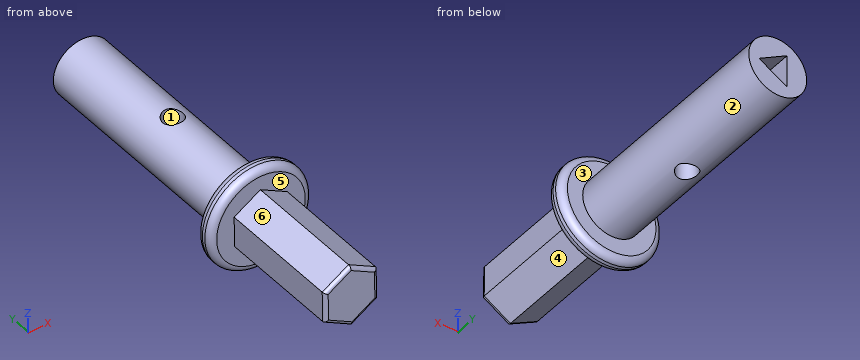
```python
from build123d import *

# Parameters (mm, degrees)
F0_R      = 4.25
F1_DEPTH  = 33
F2_DEPTH  = 6
F3_R      = 7.5
F3_R_2    = 4.25
F4_DEPTH  = 2.5
F6_DEPTH  = 18
F7_R      = 0.5
F8_R      = 1
F10_R     = 1.5
F11_DEPTH = 40


with BuildPart() as f1:
    # F0 (on Front) → F1 (new body)
    with BuildSketch(Plane.XZ):
        Circle(F0_R)
        Polygon((-1.375, 2.38157), (2.75, 0), (-1.375, -2.38157), align=None, mode=Mode.SUBTRACT)
        Polygon((-1.375, -2.38157), (2.75, 0), (-1.375, 2.38157), align=None)
    extrude(amount=F1_DEPTH)

    # F0 (on Front) → F2 (cut)
    with BuildSketch(Plane.XZ):
        Polygon((-1.375, -2.38157), (2.75, 0), (-1.375, 2.38157), align=None)
    extrude(amount=F2_DEPTH, mode=Mode.SUBTRACT)

    # F3 (on face) → F4 (join)
    with BuildSketch(Plane.XZ.offset(33)):
        Circle(F3_R)
        Circle(F3_R_2, mode=Mode.SUBTRACT)
        Circle(F3_R_2)
    extrude(amount=F4_DEPTH)

    # F5 (on face) → F6 (join)
    with BuildSketch(Plane.XZ.offset(35.5)):
        Polygon((0.076423, -4.499351), (3.934764, -2.183492), (3.858341, 2.315859), (-0.076423, 4.499351), (-3.934764, 2.183492), (-3.858341, -2.315859), align=None)
    extrude(amount=F6_DEPTH)

    # F7
    f7_edges = [f1.edges().sort_by_distance(p)[0] for p in [
        (2.005593, -53.5, -3.341421),
        (-1.890959, -53.5, -3.407605),
        (-3.896552, -53.5, -0.066184),
        (-2.005593, -53.5, 3.341421),
        (1.890959, -53.5, 3.407605),
        (3.896552, -53.5, 0.066184),
    ]]
    fillet(f7_edges, radius=F7_R)

    # F8
    f8_edges = [f1.edges().sort_by_distance(p)[0] for p in [
        (-7.5, -35.5, 0),
        (-7.5, -33, 0),
    ]]
    fillet(f8_edges, radius=F8_R)

    # F10 (on offset) → F11 (cut)
    with BuildSketch(Plane.XY.offset(25)):
        with Locations((0, -18)):
            Circle(F10_R)
    extrude(amount=-F11_DEPTH, mode=Mode.SUBTRACT)


solid = f1.part
```
Check sheet for the modelled part. Datum: model origin and axes. Units: mm. Face numbers are marked on the shaded views. A direction names the side the tool comes from. Coordinates: 2 decimals unless noted, no trailing zeros. Write each loop counter-clockwise with the first axis right and the second up, starting at its lowest first coordinate (ties: lowest second). Pieces come first, ordered by that corner, then holes. Notation, with made-up numbers: (-3, -12) -> (8, -12) arc R34 cw to (8, 22) -> close; hole circle Ø3 at (52, -15). An arc over 180 degrees is marked (long way). Use a Markdown table: item, result.
1. Sectioned sample at C-C (y = -8). Enter the section's corners in (x, z), plus the area to 3 significant figures.
Reported:
| item | result |
|---|---|
| outline | circle Ø8.5 at (0, 0) |
| area | 56.7 mm2 |
2. Release check for a two-part mould opening along X. For the marked faces 1, 2 and 3 record: pulls with the +X half, pulls with the -X half, needs draft (parallel to the pull), parting line crosses it, or undercut.
Reported:
| item | result |
|---|---|
| face 1 | undercut |
| face 2 | parting line crosses it |
| face 3 | needs draft |
3. Tool access check on the marked faces 4, 5 and 6. Record the directions out of +Z, -Z, +X, -X, +Y, -Y that give a thin tool (end or side, any length) a straight path to the whole face; none if there is none.
Reported:
| item | result |
|---|---|
| face 4 | -Z, +X, -Y |
| face 5 | -Y |
| face 6 | +Z, -X, -Y |
4. Go/stop test with flat-tipped pins: pin 1 Ø1 at (y, z) = (-31.5, 2) entering from +X; pin 2 Ø6 at (y, z) = (-23.5, 1) entering from +X; pin 3 Ø8 at (x, y) = (4.5, -33.5) entering from +Z; pin 4 Ø2 at (x, z) = (1.5, 0) entering from +Y. Record where each tip stops, or that it passes through.
Reported:
| item | result |
|---|---|
| pin 1 | stops at x = 3.98 |
| pin 2 | stops at x = 4.25 |
| pin 3 | stops at z = 7.48 |
| pin 4 | stops at y = 0 |
5. Sectioned sample at A-A (y = -42). Enter the section's corners in (x, z), plus the area to 3 significant figures.
Reported:
| item | result |
|---|---|
| outline | (-3.93, 2.18) -> (-3.86, -2.32) -> (0.08, -4.5) -> (3.93, -2.18) -> (3.86, 2.32) -> (-0.08, 4.5) -> close |
| area | 52.6 mm2 |
6. Sectioned sample at B-B (y = -18). Enter the section's corners in (x, z).
Reported:
| item | result |
|---|---|
| outline | (-1.5, -3.98) -> (-1.5, 3.98) arc R4.25 ccw to start; (1.5, -3.98) arc R4.25 ccw to (1.5, 3.98) -> close |
7. Scan lines: line 1 along Y through (x, z) = (0, -2); line 2 along Y through (x, z) = (0, 0); line 3 along Y through (x, z) = (5.5, -2.5). Record each from-to range of solid material in increasing order.
Reported:
| item | result |
|---|---|
| line 1 | y = -53.5 to -19.5, -16.5 to 0 |
| line 2 | y = -53.5 to -19.5, -16.5 to -6 |
| line 3 | y = -35.5 to -33 |
